```python
from build123d import *
from OCP.BRepFilletAPI import BRepFilletAPI_MakeChamfer

# Parameters (mm, degrees)
SKETCH1_W            = 158
SKETCH1_H            = 115
BOSS_EXTRUDE1_DEPTH  = 10
SKETCH2_W            = 148
SKETCH2_H            = 105
CUT_EXTRUDE1_DEPTH   = 2
BOSS_EXTRUDE2_DEPTH  = 1.5
SKETCH4_W            = 5
SKETCH4_H            = 10
BOSS_EXTRUDE3_DEPTH  = 38
M3_CLEARANCE_HOLE1_D = 3.4
CHAMFER3_SIZE        = 2
CHAMFER4_SIZE        = 5
CHAMFER4_SIZE_2      = 18.660254038
CHAMFER5_SIZE        = 5
CHAMFER6_SIZE        = 2


with BuildPart() as part:
    # Sketch1 → Boss-Extrude1 (new body)
    with BuildSketch(Plane.XY):
        Rectangle(SKETCH1_W, SKETCH1_H)
    extrude(amount=BOSS_EXTRUDE1_DEPTH)

    # Sketch2 → Cut-Extrude1 (cut)
    with BuildSketch(Plane(origin=(0, 0, 0), x_dir=(-1, 0, 0), z_dir=(0, 0, -1))):
        Rectangle(SKETCH2_W, SKETCH2_H)
    extrude(amount=-CUT_EXTRUDE1_DEPTH, mode=Mode.SUBTRACT)

    # Sketch3 → Boss-Extrude2 (add)
    with BuildSketch(Plane(origin=(0, 0, 0), x_dir=(-1, 0, 0), z_dir=(0, 0, -1))):
        Polygon((-74, 42.5), (-64, 52.5), (-74, 52.5), align=None)
        Polygon((74, 52.5), (74, 42.5), (64, 52.5), align=None)
        Polygon((-74, -52.5), (-74, -42.5), (-64, -52.5), align=None)
        Polygon((74, -42.5), (64, -52.5), (74, -52.5), align=None)
    extrude(amount=-BOSS_EXTRUDE2_DEPTH)

    # Sketch4 → Boss-Extrude3 (add)
    with BuildSketch(Plane.XY.offset(10)):
        with Locations((27.5, 62.5)):
            Rectangle(SKETCH4_W, SKETCH4_H)
        with Locations((-27.5, 62.5)):
            Rectangle(SKETCH4_W, SKETCH4_H)
    extrude(amount=-BOSS_EXTRUDE3_DEPTH)

    # M3 Clearance Hole1 (through all)
    with Locations(Plane(origin=(30, 0, 0), x_dir=(0, 0, -1), z_dir=(1, 0, 0))):
        with Locations((24, 63.5), (-6, 63.5)):
            Hole(M3_CLEARANCE_HOLE1_D / 2)

    # Chamfer3
    chamfer3_edges = [part.edges().sort_by_distance(p)[0] for p in [
        (-27.5, 67.5, -28),
        (27.5, 67.5, -28),
        (27.5, 67.5, 10),
        (-27.5, 67.5, 10),
    ]]
    chamfer(chamfer3_edges, length=CHAMFER3_SIZE)

    # Chamfer4
    chamfer4_edges_1 = [part.edges().sort_by_distance(p)[0] for p in [
        (-27.5, 57.5, 0),
    ]]
    chamfer4_side_1 = [part.faces().sort_by_distance(p)[0] for p in [
        (-27.5, 57.4, 0),
    ]]
    chamfer4_edges_2 = [part.edges().sort_by_distance(p)[0] for p in [
        (27.5, 57.5, 0),
    ]]
    chamfer4_side_2 = [part.faces().sort_by_distance(p)[0] for p in [
        (27.5, 57.5, -0.1),
    ]]
    chamfer4 = BRepFilletAPI_MakeChamfer(part.part.solid().wrapped)
    for e in chamfer4_edges_1:
        chamfer4.Add(CHAMFER4_SIZE - 0.0001, CHAMFER4_SIZE_2 - 0.0001, e.wrapped, chamfer4_side_1[0].wrapped)
    for e in chamfer4_edges_2:
        chamfer4.Add(CHAMFER4_SIZE_2 - 0.0001, CHAMFER4_SIZE - 0.0001, e.wrapped, chamfer4_side_2[0].wrapped)
    add(Compound.cast(chamfer4.Shape()), mode=Mode.REPLACE)  # a hair under: the kernel refuses the full size

    # Chamfer5
    chamfer5_edges = [part.edges().sort_by_distance(p)[0] for p in [
        (79, 57.5, 5),
        (-79, 57.5, 5),
        (-79, -57.5, 5),
        (79, -57.5, 5),
    ]]
    chamfer(chamfer5_edges, length=CHAMFER5_SIZE)

    # Chamfer6
    chamfer6_edges = [part.edges().sort_by_distance(p)[0] for p in [
        (-27.5, 57.5, -28),
        (27.5, 57.5, -28),
    ]]
    chamfer(chamfer6_edges, length=CHAMFER6_SIZE)


solid = part.part
```
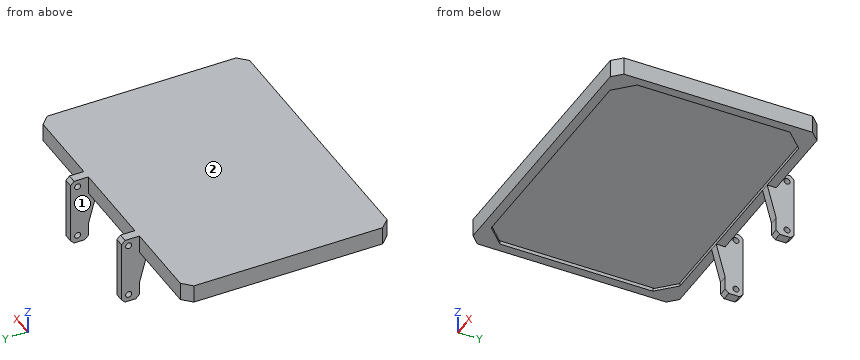
Geometry check sheet. Reference: the model listing, model coordinates, mm. Face numbers are marked on the shaded views. Give positions to 0.01 mm unless a question says otherwise; leave off trailing zeros. Loops run counter-clockwise (first coordinate to the right, second up) from the corner with the lowest first, then second, coordinate; pieces in that order, holes last. Notation, with made-up numbers: (40.5, -12) - (90.5, -12) arc R14 cw to (90.5, -6) - close; hole circle Ø4 at (8.25, -29.5). An arc over 180 degrees is marked (long way). Use CSV: the item, a comma, the result in double quotes. Start each with the question number.
Q1. Section check A-A, the plane z = -24. Record the cut outline in (x, y).
Q2. Go/stop test with flat-tipped pins: pin 1 Ø12 at (x, z) = (-41, -5) entering from +Y; pin 2 Ø4 at (y, z) = (63.5, 6) entering from -X; pin 3 Ø3 at (y, z) = (63.5, 6) entering from -X; pin 4 Ø4 at (x, z) = (-28.5, -23) entering from -Y. Record where each tip stops, or that it passes through.
Q3. Release check for a two-part mould opening along X. For the marked faces 1 and 2 record: +X half, -X half, draft (parallel to the pull), parting line (faces both ways), or undercut.
Q4. Scan lines: probe 1 along X at (y, z) = (-24.5, 1); probe 2 along Z at (x, y) = (-27, 63); probe 3 along Y at (x, z) = (-28.9, 6). Record each from-to range of solid material in increasing order. Write a range as from..to.
Q5. Section check D-D, the plane x = -55.5. Record the cut outline in (y, z).
Q6. Section check C-C, the plane z = 6. Record the cut outline in (x, y).
Q7. Section check B-B, the plane y = 63.5. Record the cut outline in (x, z).
Findings below:
1,outline,"(-30, 57.5) - (-25, 57.5) - (-25, 61.8) - (-30, 61.8) - close; (-30, 65.2) - (-25, 65.2) - (-25, 67.5) - (-30, 67.5) - close; (25, 57.5) - (30, 57.5) - (30, 61.8) - (25, 61.8) - close; (25, 65.2) - (30, 65.2) - (30, 67.5) - (25, 67.5) - close"
2,pin 1,"stops at y = 57.5"
2,pin 2,"stops at x = -30"
2,pin 3,"passes through"
2,pin 4,"stops at y = 57.5"
3,face 1,"undercut"
3,face 2,"draft"
4,probe 1,"x = -79..-74, 74..79"
4,probe 2,"z = -28..-25.62, -22.38..4.38, 7.62..10"
4,probe 3,"y = -57.5..61.8, 65.2..67.5"
5,outline,"(-57.5, 0) - (-52.5, 0) - (-52.5, 2) - (52.5, 2) - (52.5, 0) - (57.5, 0) - (57.5, 10) - (-57.5, 10) - close"
6,outline,"(-79, -52.5) - (-74, -57.5) - (74, -57.5) - (79, -52.5) - (79, 52.5) - (74, 57.5) - (30, 57.5) - (30, 61.8) - (25, 61.8) - (25, 57.5) - (-25, 57.5) - (-25, 61.8) - (-30, 61.8) - (-30, 57.5) - (-74, 57.5) - (-79, 52.5) - close; (-30, 65.2) - (-25, 65.2) - (-25, 67.5) - (-30, 67.5) - close; (25, 65.2) - (30, 65.2) - (30, 67.5) - (25, 67.5) - close"
7,outline,"(-30, -28) - (-25, -28) - (-25, -25.7) - (-30, -25.7) - close; (-30, -22.3) - (-25, -22.3) - (-25, 4.3) - (-30, 4.3) - close; (-30, 7.7) - (-25, 7.7) - (-25, 10) - (-30, 10) - close; (25, -28) - (30, -28) - (30, -25.7) - (25, -25.7) - close; (25, -22.3) - (30, -22.3) - (30, 4.3) - (25, 4.3) - close; (25, 7.7) - (30, 7.7) - (30, 10) - (25, 10) - close"
